```python
from build123d import *

# Parameters (mm, degrees)
SKETCH2_R           = 7.5
BOSS_EXTRUDE1_DEPTH = 10
SKETCH3_R           = 6
CUT_EXTRUDE1_DEPTH  = 8
DOME1_FACE_RADIUS   = 6
DOME1_HEIGHT        = 3
FILLET1_R           = 0.5


with BuildPart() as part:
    # Sketch2 → Boss-Extrude1 (new body)
    with BuildSketch(Plane(origin=(0, 0, 0), x_dir=(1, 0, 0), z_dir=(0, 1, 0))):
        with Locations(Location((0, 0, 0), (0, 0, 270))):
            Circle(SKETCH2_R)
    extrude(amount=BOSS_EXTRUDE1_DEPTH)

    # Sketch3 → Cut-Extrude1 (cut)
    with BuildSketch(Plane(origin=(0, 10, 0), x_dir=(1, 0, 0), z_dir=(0, 1, 0))):
        with Locations(Location((0, 0, 0), (0, 0, 270))):
            Circle(SKETCH3_R)
    extrude(amount=-CUT_EXTRUDE1_DEPTH, mode=Mode.SUBTRACT)

    # Dome1: an elliptical dome of height H over a round flat face of radius A is half a spheroid: the quarter ellipse of half axes A and H revolved about the face's axis
    with BuildSketch(Plane((0, 2, 0), x_dir=(0, 0, -1), z_dir=(1, 0, 0)), mode=Mode.PRIVATE) as dome1_quarter:
        Ellipse(DOME1_FACE_RADIUS, DOME1_HEIGHT)
        Rectangle(DOME1_FACE_RADIUS, DOME1_HEIGHT, align=(Align.MIN, Align.MIN), mode=Mode.INTERSECT)
    revolve(dome1_quarter.sketch, axis=Axis((0, 2, 0), (0, 1, 0)))

    # Fillet1
    fillet1_edges = [part.edges().sort_by_distance(p)[0] for p in [
        (0, 10, -7.5),
    ]]
    fillet(fillet1_edges, radius=FILLET1_R)


solid = part.part
```
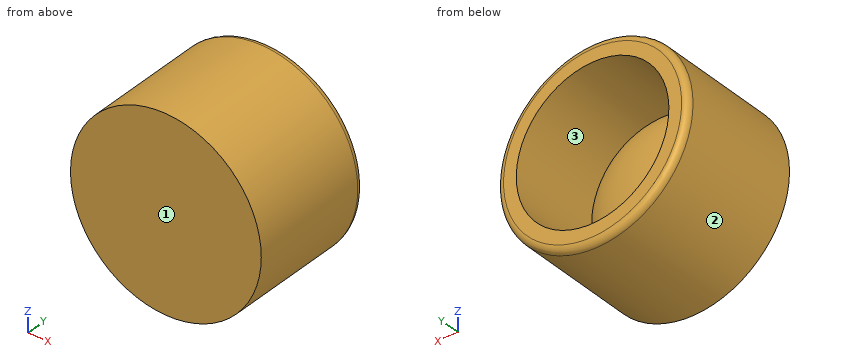
The model under review builds one solid part; all positions refer to its coordinate system, in mm. Face numbers are marked on the shaded views. Round coordinates to 2 decimals unless told otherwise and drop trailing zeros. Order: outer loops, then holes, each group sorted by start corner. A loop starts at its lowest first (then second) coordinate and runs counter-clockwise, first axis right, second up.
Item 1: Draft analysis for pull direction Z (two halves, no side actions). For the marked faces 1, 2 and 3, state which applies: released by +Z, released by -Z, zero draft, split by the parting line, or undercut.
Working result:
face 1: zero draft
face 2: split by the parting line
face 3: undercut
Item 2: To check wall thickness, follow probe 1 along X at (y, z) = (7.25, 0); probe 2 along Z at (x, y) = (-2.5, 2.75); probe 3 along Z at (x, y) = (4.5, 1.5). State the ranges of each line that lie inside material, in increasing order.
Working result:
probe 1: x = -7.5 to -6, 6 to 7.5
probe 2: z = -7.07 to -5.45, -5.24 to 5.24, 5.45 to 7.07
probe 3: z = -6 to 6
Item 3: Add section B-B, the plane y = 2.5. Count the separate pieces of the cut face and the enclosed holes in it, and give its area (3 significant figures).
Working result:
separate pieces: 2
enclosed holes: 1
area: 174 mm2
Item 4: For pin 1 (6 mm diameter, centred on y = 7, z = 3.5, fed in from +X); pin 2 (5 mm diameter, centred on x = -5, y = 8, fed in from -Z); pin 3 (5 mm diameter, centred on x = 5.5, y = 3.5, fed in from -Z), all flat-tipped, find the tip position at first contact; note any pin that passes through.
Working result:
pin 1: stops at x = 7.48
pin 2: stops at z = -7.07
pin 3: stops at z = -6.87
Item 5: Add section A-A, the plane y = 9.25. State the section outline as (x, z) points, and give its area (3 significant figures).
Working result:
outline: circle Ø15 at (0, 0); hole circle Ø12 at (0, 0)
area: 63.6 mm2
